Build history of the part. All positions in model axes, mm. Round coordinates to 2 decimals unless told otherwise and drop trailing zeros. Write each loop counter-clockwise with the first axis right and the second up, starting at its lowest first coordinate (ties: lowest second). Pieces come first, ordered by that corner, then holes. Notation, with made-up numbers: (-37, 84.25) - (-9, 84.25) arc R24 ccw to (-9, 110.25) - close; hole circle Ø3 at (18.25, 31). An arc over 180 degrees is marked (long way). Answer as a JSON object with one key per item and string values. Group by question number.
Item 1: Slice it at C-C, the plane y = -8. List the corners of the cut face in (x, z), then the cut area to 3 significant figures.
Item 2: Flat gauge pins, fed straight in: pin 1 (1.6 mm diameter, centred on x = -66, z = -0.5, fed in from +Y); pin 2 (2 mm diameter, centred on x = -64, z = -1.5, fed in from -Y). Where does each tip first touch, or does it go through?
Item 3: Slice it at A-A, the plane z = -1.45. List the corners of the cut face in (x, y).
Item 4: Probe line 1 (X direction, y = -34, z = 1.45); line 2 (X direction, y = 1, z = -1.75); line 3 (Y direction, x = 40.5, z = -0.75). List the from-to ranges inside material, lowest first. Write a range as from..to.
Item 5: Slice it at B-B, the plane x = 35.5. List the corners of the cut face in (y, z).
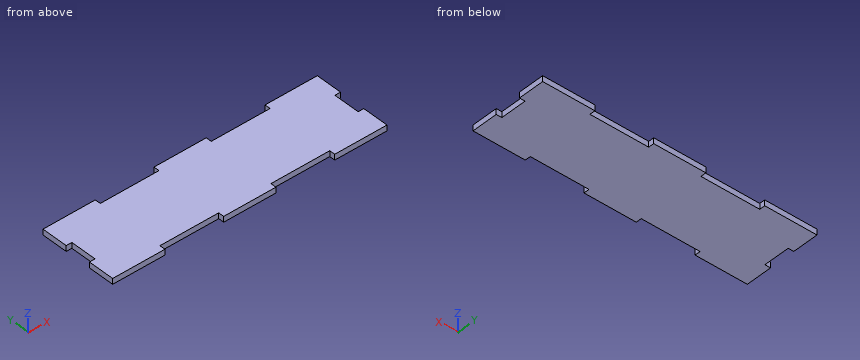
from build123d import *

# Parameters (mm, degrees)
SKETCH1_W           = 266.7
SKETCH1_H           = 76.2
BOSS_EXTRUDE1_DEPTH = 2.7305
CAVITY1_START       = -38.1
CAVITY1_OUTLINE_W   = 57.15
CAVITY1_OUTLINE_H   = 5.461
CAVITY1_DEPTH       = 5.461
CAVITY1_START_2     = 32.639
CAVITY1_2_OUTLINE_W = 57.15
CAVITY1_2_OUTLINE_H = 5.461
CAVITY1_2_DEPTH     = 5.461
SKETCH2_W           = 5.461
SKETCH2_H           = 25.4
CUT_EXTRUDE1_DEPTH  = 139.793569811


# Read off the part's stored shape, not the designer's step: Cavity1
with BuildPart() as part:
    # Sketch1 → Boss-Extrude1 (new, symmetric)
    with BuildSketch(Plane.XY):
        Rectangle(SKETCH1_W, SKETCH1_H)
    extrude(amount=BOSS_EXTRUDE1_DEPTH, both=True)

    # Cavity1 outline → Cavity1 (cut)
    with BuildSketch(Plane(origin=(0, 0, 0), x_dir=(1, 0, 0), z_dir=(0, 1, 0)).offset(CAVITY1_START)):
        with Locations((-53.975, 0)):
            Rectangle(CAVITY1_OUTLINE_W, CAVITY1_OUTLINE_H)
        with Locations((53.975, 0)):
            Rectangle(CAVITY1_OUTLINE_W, CAVITY1_OUTLINE_H)
    extrude(amount=CAVITY1_DEPTH, mode=Mode.SUBTRACT)

    # Cavity1 2 outline → Cavity1 2 (cut)
    with BuildSketch(Plane(origin=(0, 0, 0), x_dir=(1, 0, 0), z_dir=(0, 1, 0)).offset(CAVITY1_START_2)):
        with Locations((-53.975, 0)):
            Rectangle(CAVITY1_2_OUTLINE_W, CAVITY1_2_OUTLINE_H)
        with Locations((53.975, 0)):
            Rectangle(CAVITY1_2_OUTLINE_W, CAVITY1_2_OUTLINE_H)
    extrude(amount=CAVITY1_2_DEPTH, mode=Mode.SUBTRACT)

    # Sketch2 → Cut-Extrude1 (cut, through all)
    with BuildSketch(Plane.XY.offset(2.7305)):
        with Locations((-130.6195, 0)):
            Rectangle(SKETCH2_W, SKETCH2_H)
    cut_extrude1 = extrude(amount=-CUT_EXTRUDE1_DEPTH, mode=Mode.SUBTRACT)

    # Mirror1: Cut-Extrude1 across plane
    add(cut_extrude1.mirror(Plane(origin=(0, 0, 0), x_dir=(0, 0, 1), z_dir=(1, 0, 0))), mode=Mode.SUBTRACT)


solid = part.part
Geometry says:
{
 "1": {"outline": "(-127.89, -2.73) - (127.89, -2.73) - (127.89, 2.73) - (-127.89, 2.73) - close", "area": "1,400 mm^2"},
 "2": {"pin 1": "stops at y = 32.64", "pin 2": "stops at y = -32.64"},
 "3": {"outline": "(-133.35, -38.1) - (-82.55, -38.1) - (-82.55, -32.64) - (-25.4, -32.64) - (-25.4, -38.1) - (25.4, -38.1) - (25.4, -32.64) - (82.55, -32.64) - (82.55, -38.1) - (133.35, -38.1) - (133.35, -12.7) - (127.89, -12.7) - (127.89, 12.7) - (133.35, 12.7) - (133.35, 38.1) - (82.55, 38.1) - (82.55, 32.64) - (25.4, 32.64) - (25.4, 38.1) - (-25.4, 38.1) - (-25.4, 32.64) - (-82.55, 32.64) - (-82.55, 38.1) - (-133.35, 38.1) - (-133.35, 12.7) - (-127.89, 12.7) - (-127.89, -12.7) - (-133.35, -12.7) - close"},
 "4": {"line 1": "x = -133.35..-82.55, -25.4..25.4, 82.55..133.35", "line 2": "x = -127.89..127.89", "line 3": "y = -32.64..32.64"},
 "5": {"outline": "(-32.64, -2.73) - (32.64, -2.73) - (32.64, 2.73) - (-32.64, 2.73) - close"}
}
